Drawing for the job (mm, zero at the part's lowest x, y, z). A direction names the side the tool comes from. Give positions to 0.01 mm unless a question says otherwise; leave off trailing zeros. Order: outer loops, then holes, each group sorted by start corner. A loop starts at its lowest first (then second) coordinate and runs counter-clockwise, first axis right, second up. Notation, with made-up numbers: (24.25, 35) - (74.25, 35) arc R16 cw to (74.25, 66) - close; hole circle Ø11 at (22, 87.25). An arc over 180 degrees is marked (long way). One line per item, written item: value.
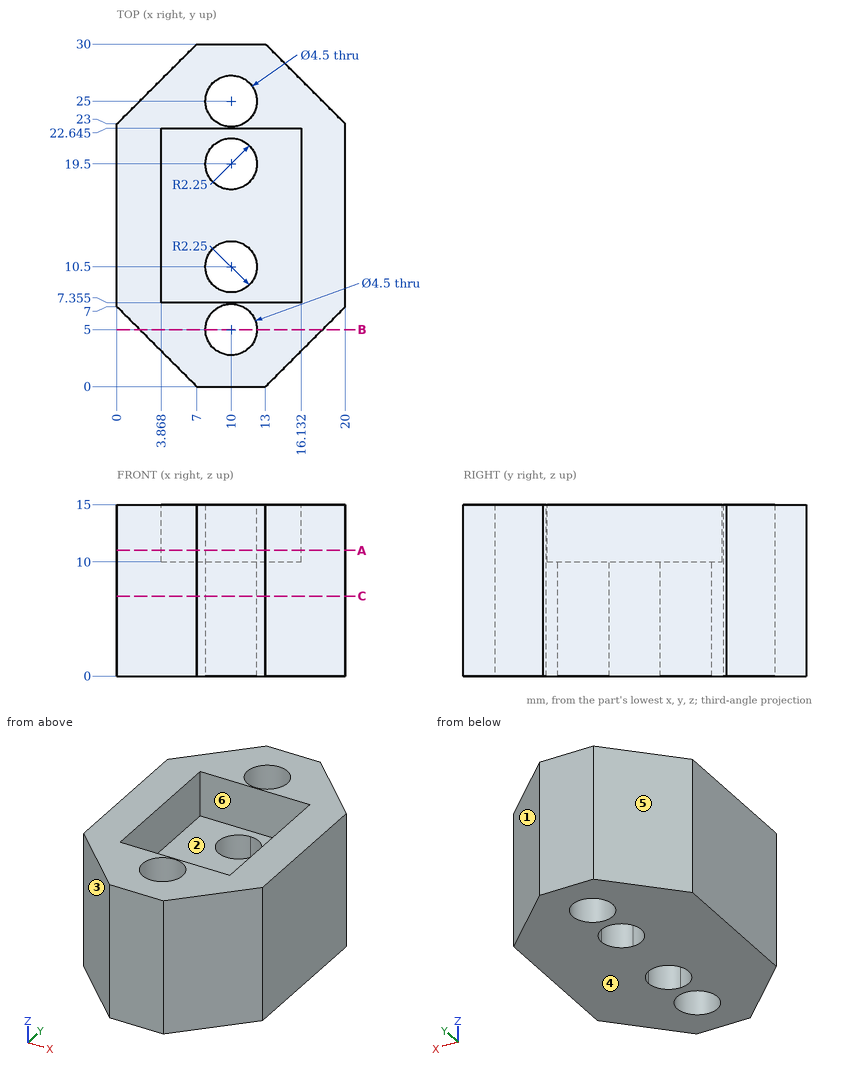
1) Cut at C-C, the plane z = 7. Give the cut face in (x, y), then the cut area to 3 significant figures.
Outcome:
outline: (0, 7) - (7, 0) - (13, 0) - (20, 7) - (20, 23) - (13, 30) - (7, 30) - (0, 23) - close; hole circle Ø4.5 at (10, 5); hole circle Ø4.5 at (10, 10.5); hole circle Ø4.5 at (10, 19.5); hole circle Ø4.5 at (10, 25)
area: 438 mm^2
2) Mould opens along Y. For the marked faces 1, 2, 3 and 4 say: released by +Y, released by -Y, zero draft, split by the parting line, or undercut.
Outcome:
face 1: released by +Y
face 2: undercut
face 3: released by -Y
face 4: zero draft
3) Pin check, flat tips, straight feed: pin 1 (3.5 mm diameter, centred on x = 9.5, y = 15.5, fed in from +Z); pin 2 (3 mm diameter, centred on x = 3, z = 6.5, fed in from -Y); pin 3 (1 mm diameter, centred on y = 3, z = 12, fed in from +X). Stop position of each tip, or through.
Outcome:
pin 1: stops at z = 10
pin 2: stops at y = 2.5
pin 3: stops at x = 16.5
4) Drill centre lines: line 1 along Y through (x, z) = (10, 5); line 2 along Y through (x, z) = (11.5, 8.5); line 3 along Y through (x, z) = (12, 12) (1 decimal). Where is each one in solid material? Low to high. Write a range as from..to.
Outcome:
line 1: y = 0..2.75, 7.25..8.25, 12.75..17.25, 21.75..22.75, 27.25..30
line 2: y = 0..3.32, 6.68..8.82, 12.18..17.82, 21.18..23.32, 26.68..30
line 3: y = 0..4, 6..7.4, 22.6..24, 26..30
5) Cut at B-B, the plane y = 5. Give the cut face in (x, z).
Outcome:
outline: (2, 0) - (7.75, 0) - (7.75, 15) - (2, 15) - close; (12.25, 0) - (18, 0) - (18, 15) - (12.25, 15) - close
6) Cut at A-A, the plane z = 11. Give the number of separate pieces and of enclosed holes in the cut face, then the cut area to 3 significant figures.
Outcome:
separate pieces: 1
enclosed holes: 3
area: 283 mm^2
7) Which spindle directions (+Z, -Z, +X, -X, +Y, -Y) get a long thin tool onto all of the face, cutting with end or side? Do the marked faces 5 and 6. Say none if no direction does.
Outcome:
face 5: +Z, -Z, -X, +Y
face 6: +Z
